The model under review builds one solid part; all positions refer to its coordinate system, in mm. A direction names the side the tool comes from. Coordinates: 2 decimals unless noted, no trailing zeros. Write each loop counter-clockwise with the first axis right and the second up, starting at its lowest first coordinate (ties: lowest second). Pieces come first, ordered by that corner, then holes. Notation, with made-up numbers: (43.25, 11.25) - (66.25, 11.25) arc R22 cw to (66.25, 37.25) - close; hole circle Ø5 at (45.5, 80). An arc over 180 degrees is marked (long way). Put each result on its own line as item: value. Start each with the question number.
Item 1: For pin 1 (5 mm diameter, centred on x = -29, z = 10.5, fed in from +Y); pin 2 (7.5 mm diameter, centred on y = 13.5, z = 5.5, fed in from -X); pin 3 (6 mm diameter, centred on x = -30.5, y = -29.5, fed in from +Z); pin 4 (10 mm diameter, centred on y = -27.5, z = 9, fed in from +X), all flat-tipped, find the tip position at first contact; note any pin that passes through.
Item 2: Consider section B-B on z = 4.5. Give the boundary of the cut face in (x, y).
Item 3: Machinability: for faces 1 (the face through (-42.39, 12.52, 0.15)), 2 (the face through (-43, 13, 14.526)), 3 (the face through (-45.397, -31.661, 0.038)), 4 (the face through (-50.928, 13, 0)), which of the approach directions +Z, -Z, +X, -X, +Y, -Y give a long, thin tool a straight path to every point of the face, cutting with its end or side? Answer none if there is none.
Item 4: To check wall thickness, follow L1, parallel to Y at x = -13, z = -9.5; L2, parallel to Z at x = -38.5, y = -10; L3, parallel to Z at x = -49, y = -35. State the ranges of each line that lie inside material, in increasing order. Write a range as [from, to].
Item 5: Consider section A-A on x = -40. Give the boundary of the cut face in (y, z).
Item 6: Consider section D-D on y = -34. Give the boundary of the cut face in (x, z), then the cut area to 3 significant figures.
Item 7: Consider section C-C on y = -7.5. Give the boundary of the cut face in (x, z), then the cut area to 3 significant figures.
```python
from build123d import *

# Parameters (mm, degrees)
F2_DEPTH = 25.4
F4_DEPTH = 12.7
F7_DEPTH = 25.4


with BuildPart() as f2:
    # F1 (on Front) → F2 (new body)
    with BuildSketch(Plane.XZ):
        Polygon((5.1933536553, 14.8594833362), (-51.9565972747, 14.9343745474), (-51.9565972747, -14.4059932236), (5.1933536553, -16.8905166638), align=None)
    extrude(amount=F2_DEPTH)

    # F3 (on face) + F2_face1 (on face) → F4 (join)
    with BuildSketch(Plane.XZ.offset(25.4)):
        Polygon((-51.3677446578, -14.4315928628), (-39.2566081791, 14.917732056), (-51.9565972747, 14.9343745474), (-51.9565972747, -14.4059932236), align=None)
    with BuildSketch(Plane(origin=(-23.0059205639, 0, -0.3840757402), x_dir=(1, 0, 0), z_dir=(0, 1, 0))):
        Polygon((28.1992742193, -15.2435590764), (28.1992742193, 16.5064409236), (-28.9506767108, 14.0219174834), (-28.9506767108, -15.3184502876), align=None)
    extrude(amount=F4_DEPTH, dir=(0, -1, 0))

    # F6 (on face) → F7 (join)
    with BuildSketch(Plane(origin=(0, 0, 0), x_dir=(-1, 0, 0), z_dir=(0, 1, 0))):
        Polygon((34.0825431049, 14.5258735865), (50.9283207357, -14.6334338933), (50.9283207357, 14.5258735865), align=None)
    extrude(amount=F7_DEPTH)


solid = f2.part
```
Report:
1. pin 1: y = 0
1. pin 2: x = -50.93
1. pin 3: through
1. pin 4: x = 5.19
2. outline: (-51.96, -38.1) - (-43.56, -38.1) - (-43.56, -25.4) - (5.19, -25.4) - (5.19, 0) - (-39.87, 0) - (-39.87, 25.4) - (-50.93, 25.4) - (-50.93, 0) - (-51.96, 0) - close
3. face 1: -Z, +X, +Y
3. face 2: +Z, +X, -X, +Y
3. face 3: -Z, +X, -Y
3. face 4: +Z, -Z, -X, +Y
4. L1: [-25.4, 0]
4. L2: [-14.99, 14.92]
4. L3: [-8.69, 14.93]
5. outline: (-38.1, 13.12) - (-25.4, 13.12) - (-25.4, -14.93) - (0, -14.93) - (0, 4.28) - (25.4, 4.28) - (25.4, 14.53) - (0, 14.53) - (0, 14.92) - (-38.1, 14.92) - close
6. outline: (-51.96, -14.41) - (-51.37, -14.43) - (-39.26, 14.92) - (-51.96, 14.93) - close
6. area: 195 mm²
7. outline: (-51.96, -14.41) - (5.19, -16.89) - (5.19, 14.86) - (-51.96, 14.93) - close
7. area: 1,750 mm²
